For this review, use the dimensioned drawing (mm, ordinates from the lowest corner) and the shaded views. Give positions to 0.01 mm unless a question says otherwise; leave off trailing zeros. Loops run counter-clockwise (first coordinate to the right, second up) from the corner with the lowest first, then second, coordinate; pieces in that order, holes last. Notation, with made-up numbers: (66.5, 73.25) - (109.5, 73.25) arc R18 cw to (109.5, 84.25) - close; hole circle Ø6 at (-27, 5.25). An arc over 180 degrees is marked (long way). Put each result on its own line as item: value.
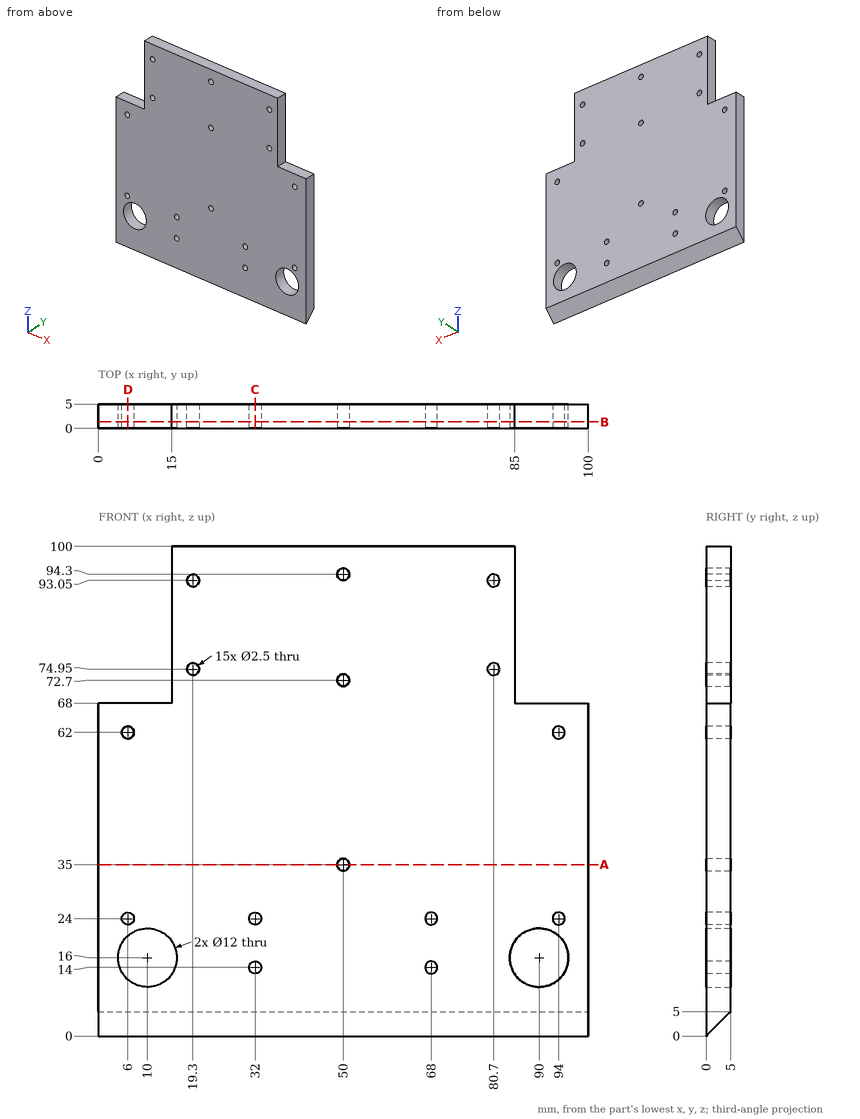
1) Take a section at B-B on y = 1.35. State how many separate pieces and enclosed holes the cut face has, and give its area (3 significant figures).
Geometry check:
separate pieces: 1
enclosed holes: 17
area: 8,610 mm²
2) Take a section at A-A on z = 35. State the section outline as (x, y) points.
Geometry check:
outline: (0, 0) - (48.75, 0) - (48.75, 5) - (0, 5) - close; (51.25, 0) - (100, 0) - (100, 5) - (51.25, 5) - close
3) Insertion check: pin 1 Ø2.5 at (y, z) = (2, 89) entering from +X; pin 2 Ø3 at (x, z) = (6, 62) entering from -Y; pin 3 Ø2 at (x, z) = (19.3, 93.05) entering from +Y. Each pin has a flat end and moves straight along its axis. Give the tip position at first contact, or say it passes through.
Geometry check:
pin 1: stops at x = 85
pin 2: stops at y = 0
pin 3: passes through
4) Take a section at C-C on x = 32. State the section outline as (y, z) points, and give its area (4 significant figures).
Geometry check:
outline: (0, 0) - (5, 5) - (5, 12.75) - (0, 12.75) - close; (0, 15.25) - (5, 15.25) - (5, 22.75) - (0, 22.75) - close; (0, 25.25) - (5, 25.25) - (5, 100) - (0, 100) - close
area: 462.5 mm²
5) Wall thickness on line 1 (X direction, y = 1.8, z = 74.95); line 2 (Z direction, x = 50, y = 2.45); line 3 (X direction, y = 3.8, z = 72.7): over which ranges is each line inside the solid? List them lowest first.
Geometry check:
line 1: x = 15 to 18.05, 20.55 to 79.45, 81.95 to 85
line 2: z = 2.45 to 33.75, 36.25 to 71.45, 73.95 to 93.05, 95.55 to 100
line 3: x = 15 to 48.75, 51.25 to 85
6) Take a section at D-D on x = 6. State the section outline as (y, z) points.
Geometry check:
outline: (0, 0) - (5, 5) - (5, 11.53) - (0, 11.53) - close; (0, 20.47) - (5, 20.47) - (5, 22.75) - (0, 22.75) - close; (0, 25.25) - (5, 25.25) - (5, 60.75) - (0, 60.75) - close; (0, 63.25) - (5, 63.25) - (5, 68) - (0, 68) - close
